Source: CAD feature listing. Evaluate the final solid. Frame: model axes, mm. A direction names the side the tool comes from. Give positions to 0.01 mm unless a question says otherwise; leave off trailing zeros. Order: outer loops, then holes, each group sorted by start corner. A loop starts at its lowest first (then second) coordinate and runs counter-clockwise, first axis right, second up. Notation, with made-up numbers: (81, 39.25) -> (115, 39.25) arc R35 ccw to (115, 77.25) -> close; hole circle Ø10 at (4, 44). An arc over 180 degrees is marked (long way). Answer in a Markdown table with one row per item.
```python
from build123d import *

# Parameters (mm, degrees)
SKETCH1_W           = 80
SKETCH1_H           = 80
SKETCH1_W_2         = 50
SKETCH1_H_2         = 50
BOSS_EXTRUDE1_DEPTH = 150
SKETCH2_R           = 5
CUT_EXTRUDE1_DEPTH  = 5


with BuildPart() as part:
    # Sketch1 → Boss-Extrude1 (new body)
    with BuildSketch(Plane.XY):
        Rectangle(SKETCH1_W, SKETCH1_H)
        Rectangle(SKETCH1_W_2, SKETCH1_H_2, mode=Mode.SUBTRACT)
    extrude(amount=BOSS_EXTRUDE1_DEPTH)

    # Sketch2 → Cut-Extrude1 (cut)
    with BuildSketch(Plane.ZY.offset(40)):
        with Locations(Location((75, 0, 0), (0, 0, 270))):
            Circle(SKETCH2_R)
    extrude(amount=-CUT_EXTRUDE1_DEPTH, mode=Mode.SUBTRACT)


solid = part.part
```
(1) Section query A-A (y = 21.5). Return the cut outline in (x, z).
A:
| item | result |
|---|---|
| outline | (-40, 0) -> (-25, 0) -> (-25, 150) -> (-40, 150) -> close; (25, 0) -> (40, 0) -> (40, 150) -> (25, 150) -> close |
(2) Ray query, probe 1 along X at (y, z) = (-2.5, 74.5); probe 2 along Z at (x, y) = (-36.75, 0); probe 3 along X at (y, z) = (20, 141). Return the intervals inside material, ascending.
A:
| item | result |
|---|---|
| probe 1 | x = -35 to -25, 25 to 40 |
| probe 2 | z = 0 to 70, 80 to 150 |
| probe 3 | x = -40 to -25, 25 to 40 |
(3) First-contact query: pin 1 Ø5 at (y, z) = (1, 77) entering from -X. Flat tip, straight axial feed; report the tip coordinate or a pass-through.
A:
| item | result |
|---|---|
| pin 1 | stops at x = -35 |
(4) Pull-direction query (X, two-part tool) for faces 4 (the flat face through (0, -25, 74)), 5 (the flat face through (-1, -40, 74)), 6 (the flat face through (-40, 8, 74)), 7 (the flat face through (0, 25, 74)); classes: +X half, -X half, draft (parallel to the pull), parting line (faces both ways), or undercut.
A:
| item | result |
|---|---|
| face 4 | undercut |
| face 5 | draft |
| face 6 | -X half |
| face 7 | undercut |
(5) Section query B-B (z = 94.5). Return the cut outline in (x, y).
A:
| item | result |
|---|---|
| outline | (-40, -40) -> (40, -40) -> (40, 40) -> (-40, 40) -> close; hole (-25, -25) -> (25, -25) -> (25, 25) -> (-25, 25) -> close |
(6) Access query for faces 1 (the flat face through (40, -1, 74)), 2 (the flat face through (25, 0, 74)), 3 (the cylindrical face through (-37.53, 1.08, 70.12)). Directions: +Z, -Z, +X, -X, +Y, -Y. A direction counts if a zero-diameter tool reaches every point of the face in a straight line with its end or side. Return the directions, or none.
A:
| item | result |
|---|---|
| face 1 | +Z, -Z, +X, +Y, -Y |
| face 2 | +Z, -Z |
| face 3 | -X |
(7) Section query D-D (y = 0). Return the cut outline in (x, z).
A:
| item | result |
|---|---|
| outline | (-40, 0) -> (-25, 0) -> (-25, 150) -> (-40, 150) -> (-40, 80) -> (-35, 80) -> (-35, 70) -> (-40, 70) -> close; (25, 0) -> (40, 0) -> (40, 150) -> (25, 150) -> close |
